Geometry check sheet. Reference: the model listing, model coordinates, mm. A direction names the side the tool comes from. Round coordinates to 2 decimals unless told otherwise and drop trailing zeros. Order: outer loops, then holes, each group sorted by start corner. A loop starts at its lowest first (then second) coordinate and runs counter-clockwise, first axis right, second up. Notation, with made-up numbers: M 30,22.5 L 81,22.5 A13 cw 81,47.5 Z; hole C 14,35 d10. An arc over 180 degrees is marked long. Return JSON: item names as keys, results as strings. Group by question number.
```python
from build123d import *

# Parameters (mm, degrees)
F3_DEPTH = 4.7625
F5_D     = 5.1054


with BuildPart() as f1:
    # F0 (on Right) → F1 (revolve)
    with BuildSketch(Plane.YZ):
        Polygon((-9.525, 0), (0, 0), (0, 3.175), (-9.525, 3.175), (-9.525, 6.35), (-11.1125, 6.35), (-11.1125, 7.9375), (-9.525, 7.9375), (-9.525, 11.1125), (-12.7, 11.1125), (-12.7, 7.9375), (-12.7, 6.35), (-12.7, 0), align=None)
    revolve(axis=Axis((0, 0, 5.3960988298), (0, 0, 1)))

    # F2 (on face) → F3 (cut)
    with BuildSketch(Plane.XY.offset(11.1125)):
        Polygon((0, 9.4918694648), (0.79375, 9.4918694648), (0.79375, 11.1125), (0, 11.1125), (-0.79375, 11.1125), (-0.79375, 9.4918694648), align=None)
        Polygon((0.79375, -11.1125), (0.79375, -9.4918694648), (0, -9.4918694648), (-0.79375, -9.4918694648), (-0.79375, -11.1125), (0, -11.1125), align=None)
    extrude(amount=-F3_DEPTH, mode=Mode.SUBTRACT)

    # F5 (through all)
    with Locations(Plane(origin=(0, 0, 0), x_dir=(1, 0, 0), z_dir=(0, 0, -1))):
        with Locations((0, 0)):
            Hole(F5_D / 2)


solid = f1.part
```
Q1. Material ranges on line 1 along X through (y, z) = (0, 4.9) (3 decimals); line 2 along Z through (x, y) = (-2, 4) (3 decimals); line 3 along X through (y, z) = (-4, 3.75), recorded low to high.
Q2. Section check D-D on x = 10.5. Record the cut outline in (y, z), plus the area to 3 significant figures.
Q3. Depth check by flat-ended pin: pin 1 Ø1.8 at (y, z) = (10.5, 8.5) entering from -X; pin 2 Ø3 at (x, z) = (-8.5, 5.5) entering from +Y; pin 3 Ø11.5 at (x, y) = (-5.5, 1) entering from -Z; pin 4 Ø6 at (y, z) = (-8, 7.5) entering from +X. Enter the tip coordinate at first touch or a pass-through.
Q4. Set-up check for faces 5 (the face through (-12.4, 2.75, 5.48)), 6 (the face through (10, -1, 7.938)), 7 (the face through (-5.796, 7.559, 4.785)): record each of +Z, -Z, +X, -X, +Y, -Y from which the full face is reachable in a straight line by a thin tool's end or side.
Q5. Release check for a two-part mould opening along Z. For faces 1 (the face through (-0.794, -10, 9)), 2 (the face through (11.11, -0.23, 7.15)), 3 (the face through (8.3, -5, 6.35)), 4 (the face through (-2, 2, 3.175)) record: +Z half, -Z half, draft (parallel to the pull), parting line (faces both ways), or undercut.
Geometry check:
{
 "1": {"line 1": "x = -12.7 to -9.525, 9.525 to 12.7", "line 2": "z = 0 to 3.175", "line 3": "x = -12.05 to -8.64, 8.64 to 12.05"},
 "2": {"outline": "M -7.14,0 L 7.14,0 L 7.14,11.11 L -7.14,11.11 Z; hole M -3.64,6.35 L 3.64,6.35 L 3.64,7.94 L -3.64,7.94 Z", "area": "147 mm^2"},
 "3": {"pin 1": "stops at x = -8.31", "pin 2": "stops at y = 10.6", "pin 3": "stops at z = 0", "pin 4": "stops at x = 11.67"},
 "4": {"face 5": "+Z, -Z", "face 6": "none", "face 7": "+Z"},
 "5": {"face 1": "draft", "face 2": "undercut", "face 3": "undercut", "face 4": "+Z half"}
}
